CAD build for the part. Positions are in the model's coordinates, mm. Face numbers are marked on the shaded views. Coordinates: 2 decimals unless noted, no trailing zeros. Order: outer loops, then holes, each group sorted by start corner. A loop starts at its lowest first (then second) coordinate and runs counter-clockwise, first axis right, second up. Notation, with made-up numbers: M 60,57.5 L 83,57.5 A17 ccw 83,70.5 Z; hole C 23.5,-34.5 d6. An arc over 180 degrees is marked long. Write item = value, one per line.
Solid Edge part; units mm, degrees
sketch "Sketch1" plane through (0, 0, 0) normal (0, 0, 1) x (1, 0, 0)
  line L0 (-4, -17) -> (4, -17)
  line L1 (4, -17) -> (4, 17)
  line L2 (4, 17) -> (-4, 17)
  line L3 (-4, 17) -> (-4, -17)
  circle A0 centre (0, -13) radius 1.7
  circle A1 centre (0, 13) radius 1.7
extrude "Protrusion1" add sketch "Sketch1" along normal blind 2
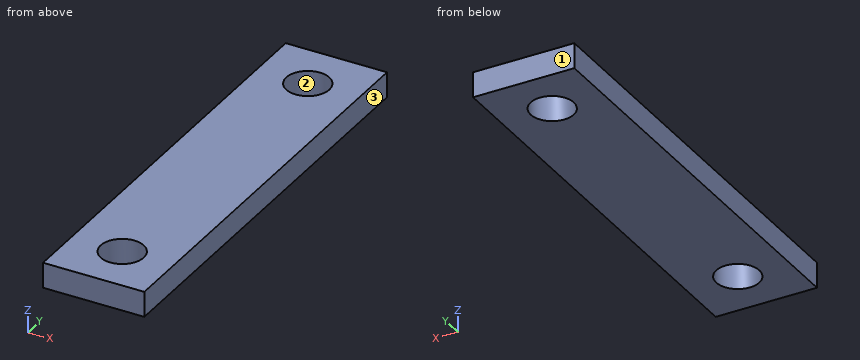
(1) Slice it at A-A, the plane x = 0. Write the cut outline in (y, z).
Evaluation:
outline = M -17,0 L -14.7,0 L -14.7,2 L -17,2 Z; M -11.3,0 L 11.3,0 L 11.3,2 L -11.3,2 Z; M 14.7,0 L 17,0 L 17,2 L 14.7,2 Z
(2) Slice it at C-C, the plane z = 1.65. Write the cut outline in (x, y).
Evaluation:
outline = M -4,-17 L 4,-17 L 4,17 L -4,17 Z; hole C 0,-13 d3.4; hole C 0,13 d3.4
(3) Slice it at B-B, the plane y = -13. Write the cut outline in (x, z), then the cut area to 3 significant figures.
Evaluation:
outline = M -4,0 L -1.7,0 L -1.7,2 L -4,2 Z; M 1.7,0 L 4,0 L 4,2 L 1.7,2 Z
area = 9.20 mm²
(4) Wall check: line 1 (Y direction, x = 0, z = 0.7); line 2 (Y direction, x = 0.5, z = 1); line 3 (X direction, y = -11.5, z = 1.85). Give the ranges that are in metal, low to high. Write a range as from..to.
Evaluation:
line_1 = -17..-14.7, -11.3..11.3, 14.7..17
line_2 = -17..-14.62, -11.38..11.38, 14.62..17
line_3 = -4..-0.8, 0.8..4
(5) Pull direction X, two halves, no side cores. Call the marked faces 1, 2 and 3: +X half, -X half, draft (parallel to the pull), parting line (faces both ways), or undercut.
Evaluation:
face_1 = draft
face_2 = undercut
face_3 = +X half
